from build123d import *

# Parameters (mm, degrees)
SKETCH1_W               = 20
SKETCH1_H               = 40
BOSS_EXTRUDE1_DEPTH     = 3
SKETCH2_W               = 2.5
SKETCH2_H               = 27
CUT_EXTRUDE1_DEPTH      = 3
SKETCH3_R               = 1.6
CUT_EXTRUDE2_DEPTH      = 1
CUT_EXTRUDE2_DEPTH_BACK = 4
SKETCH4_W               = 5
SKETCH4_H               = 27
CUT_EXTRUDE3_DEPTH      = 1
CUT_EXTRUDE3_DEPTH_BACK = 4


with BuildPart() as part:
    # Sketch1 → Boss-Extrude1 (new body)
    with BuildSketch(Plane(origin=(0, 0, 0), x_dir=(1, 0, 0), z_dir=(0, 1, 0))):
        with Locations((10, 20)):
            Rectangle(SKETCH1_W, SKETCH1_H)
    extrude(amount=BOSS_EXTRUDE1_DEPTH)

    # Sketch2 → Cut-Extrude1 (cut)
    with BuildSketch(Plane(origin=(0, 3, 0), x_dir=(1, 0, 0), z_dir=(0, 1, 0))):
        with Locations((1.25, 13.5)):
            Rectangle(SKETCH2_W, SKETCH2_H)
    cut_extrude1 = extrude(amount=-CUT_EXTRUDE1_DEPTH, mode=Mode.SUBTRACT)

    # Mirror1: Cut-Extrude1 across plane
    add(cut_extrude1.mirror(Plane.ZY.offset(-10)), mode=Mode.SUBTRACT)

    # Sketch3 → Cut-Extrude2 (cut, two sides)
    with BuildSketch(Plane(origin=(0, 3, 0), x_dir=(1, 0, 0), z_dir=(0, 1, 0))) as cut_extrude2_sk:
        with Locations((10, 33.5)):
            Circle(SKETCH3_R)
    extrude(amount=CUT_EXTRUDE2_DEPTH, mode=Mode.SUBTRACT)
    extrude(cut_extrude2_sk.sketch, amount=-CUT_EXTRUDE2_DEPTH_BACK, mode=Mode.SUBTRACT)

    # Sketch4 → Cut-Extrude3 (cut, two sides)
    with BuildSketch(Plane(origin=(0, 3, 0), x_dir=(1, 0, 0), z_dir=(0, 1, 0))) as cut_extrude3_sk:
        with Locations((10, 13.5)):
            Rectangle(SKETCH4_W, SKETCH4_H)
    extrude(amount=CUT_EXTRUDE3_DEPTH, mode=Mode.SUBTRACT)
    extrude(cut_extrude3_sk.sketch, amount=-CUT_EXTRUDE3_DEPTH_BACK, mode=Mode.SUBTRACT)


solid = part.part
Build history of the part. All positions in model axes, mm. A direction names the side the tool comes from. Coordinates: 2 decimals unless noted, no trailing zeros. Order: outer loops, then holes, each group sorted by start corner. A loop starts at its lowest first (then second) coordinate and runs counter-clockwise, first axis right, second up. Notation, with made-up numbers: M 24.5,44.5 L 36.5,44.5 A23 ccw 36.5,63.5 Z; hole C 36.5,-21 d11. An arc over 180 degrees is marked long. One line per question, with ' | ' between items. Start each with the question number.
Q1. Saw through at B-B (x = 10). List the corners of the cut face in (y, z).
Q2. Saw through at C-C (y = 2.45). List the corners of the cut face in (x, z), then the cut area to 3 significant figures.
Q3. Probe L1, parallel to X at y = 1.8, z = -33.5; L2, parallel to Z at x = 10, y = 1.7; L3, parallel to X at y = 1.55, z = -11.5. List the from-to ranges inside material, lowest first. Write a range as from..to.
Q4. 3-axis set-ups, long thin cutter, end or side, ignore diameter. For faces 5 (the face through (2.5, 2, -13)), 6 (the face through (19, 2, -27)), 7 (the face through (12.5, 2, -13)), 8 (the face through (5, 0, -25)): which of +Z, -Z, +X, -X, +Y, -Y reach the whole face in a straight line?
Q5. Saw through at A-A (z = -33.5). List the corners of the cut face in (x, y), then the cut area to 3 significant figures.
Q6. Two-plate mould, pull along X, no slides. Class faces 1 (the face through (17.5, 2, -13)), 2 (the face through (15, 1, 0)), 3 (the face through (7.5, 2, -13)), 4 (the face through (9.65, 1.52, -31.94)): +X half, -X half, draft (parallel to the pull), parting line (faces both ways), or undercut.
Q7. Flat gauge pins, fed straight in: pin 1 Ø0.8 at (x, y) = (1.5, 1) entering from +Z; pin 2 Ø0.9 at (y, z) = (2, -14.5) entering from +X; pin 3 Ø0.9 at (y, z) = (2, -11) entering from -X; pin 4 Ø6 at (x, z) = (5, -14.5) entering from -Y. Where does each tip first touch, or does it go through?
Check values:
1) outline: M 0,-40 L 3,-40 L 3,-35.1 L 0,-35.1 Z; M 0,-31.9 L 3,-31.9 L 3,-27 L 0,-27 Z
2) outline: M 0,-40 L 20,-40 L 20,-27 L 17.5,-27 L 17.5,0 L 12.5,0 L 12.5,-27 L 7.5,-27 L 7.5,0 L 2.5,0 L 2.5,-27 L 0,-27 Z; hole C 10,-33.5 d3.2 | area: 522 mm2
3) L1: x = 0..8.4, 11.6..20 | L2: z = -40..-35.1, -31.9..-27 | L3: x = 2.5..7.5, 12.5..17.5
4) face 5: +Z, -X, +Y, -Y | face 6: +Z, +X, +Y, -Y | face 7: +Z, +Y, -Y | face 8: +Z, -Z, +X, -X, -Y
5) outline: M 0,0 L 8.4,0 L 8.4,3 L 0,3 Z; M 11.6,0 L 20,0 L 20,3 L 11.6,3 Z | area: 50.4 mm2
6) face 1: +X half | face 2: draft | face 3: undercut | face 4: undercut
7) pin 1: stops at z = -27 | pin 2: stops at x = 17.5 | pin 3: stops at x = 2.5 | pin 4: stops at y = 0
